```python
from build123d import *

# Parameters (mm, degrees)
REDONDEO1_R                            = 5
CORTAR_EXTRUIR1_REACH                  = 110.669
CORTAR_EXTRUIR1_END_RADIUS             = 20
CROQUIS2_W                             = 5
CROQUIS2_H                             = 30
CORTAR_EXTRUIR1_DIRECTION_2_REACH      = 110.669
CORTAR_EXTRUIR1_DIRECTION_2_END_RADIUS = 20
CORTAR_EXTRUIR3_REACH                  = 117.3
CORTAR_EXTRUIR3_END_RADIUS             = 9
CROQUIS3_R                             = 5


with BuildPart() as part:
    # Croquis1 → Revolución1 (revolve)
    with BuildSketch(Plane(origin=(0, 0, 0), x_dir=(1, 0, 0), z_dir=(0, 1, 0))):
        Polygon((25, 0), (42, 0), (42, 6), (31, 6), (31, 36), (20, 36), (20, 91), (9, 91), (9, 25), (25, 25), align=None)
    revolve(axis=Axis((0, 0, 3.677633668), (0, 0, -1)))

    # Redondeo1
    redondeo1_edges = [part.edges().sort_by_distance(p)[0] for p in [
        (-25, 0, -25),
        (-20, 0, -36),
        (-31, 0, -6),
    ]]
    fillet(redondeo1_edges, radius=REDONDEO1_R)

    # Cortar-Extruir1: up to this cylinder (the profile starts inside it)
    cortar_extruir1_end = Plane(origin=(0, 0, -66), z_dir=(0, 0, 1)) * Cylinder(CORTAR_EXTRUIR1_END_RADIUS, 262.338, mode=Mode.PRIVATE)
    # Croquis2 → Cortar-Extruir1 (cut, up to the surface)
    with BuildSketch(Plane(origin=(0, 0, 0), x_dir=(1, 0, 0), z_dir=(0, 1, 0)), mode=Mode.PRIVATE) as cortar_extruir1_sk1:
        with Locations((17.5, 66)):
            Rectangle(CROQUIS2_W, CROQUIS2_H)
    cortar_extruir1_tool1 = extrude(cortar_extruir1_sk1.sketch, amount=-CORTAR_EXTRUIR1_REACH, mode=Mode.PRIVATE) & cortar_extruir1_end
    cortar_extruir1 = cortar_extruir1_tool1.solids().sort_by_distance((17.5, 0, -66))[0]
    add(cortar_extruir1, mode=Mode.SUBTRACT)

    # Cortar-Extruir1 direction 2: up to this cylinder (the profile starts inside it)
    cortar_extruir1_direction_2_end = Plane(origin=(0, 0, -66), z_dir=(0, 0, 1)) * Cylinder(CORTAR_EXTRUIR1_DIRECTION_2_END_RADIUS, 262.338, mode=Mode.PRIVATE)
    # Croquis2 → Cortar-Extruir1 direction 2 (cut, up to the surface)
    with BuildSketch(Plane(origin=(0, 0, 0), x_dir=(1, 0, 0), z_dir=(0, 1, 0)), mode=Mode.PRIVATE) as cortar_extruir1_direction_2_sk1:
        with Locations((17.5, 66)):
            Rectangle(CROQUIS2_W, CROQUIS2_H)
    cortar_extruir1_direction_2_tool1 = extrude(cortar_extruir1_direction_2_sk1.sketch, amount=CORTAR_EXTRUIR1_DIRECTION_2_REACH, mode=Mode.PRIVATE) & cortar_extruir1_direction_2_end
    cortar_extruir1_direction_2 = cortar_extruir1_direction_2_tool1.solids().sort_by_distance((17.5, 0, -66))[0]
    add(cortar_extruir1_direction_2, mode=Mode.SUBTRACT)
    cortar_extruir1 = cortar_extruir1 + cortar_extruir1_direction_2  # both directions under the feature's name, for the pattern or mirror that repeats it

    # Cortar-Extruir3: up to this cylinder (the profile starts outside it)
    cortar_extruir3_end = Plane(origin=(0, 0, -66), z_dir=(0, 0, 1)) * Cylinder(CORTAR_EXTRUIR3_END_RADIUS, 253.6, mode=Mode.PRIVATE)
    # Croquis3 → Cortar-Extruir3 (cut, up to the surface)
    with BuildSketch(Plane(origin=(15, 0, 0), x_dir=(0, 0, -1), z_dir=(1, 0, 0)), mode=Mode.PRIVATE) as cortar_extruir3_sk1:
        with Locations((66, 0)):
            Circle(CROQUIS3_R)
    cortar_extruir3_tool1 = extrude(cortar_extruir3_sk1.sketch, amount=-CORTAR_EXTRUIR3_REACH, mode=Mode.PRIVATE) - cortar_extruir3_end
    cortar_extruir3 = cortar_extruir3_tool1.solids().sort_by_distance((15, 0, -66))[0]
    add(cortar_extruir3, mode=Mode.SUBTRACT)

    # Simetría2: Cortar-Extruir1, Cortar-Extruir3 across plane
    add(cortar_extruir1.mirror(Plane(origin=(0, 0, 0), x_dir=(0, 0, 1), z_dir=(1, 0, 0))), mode=Mode.SUBTRACT)
    add(cortar_extruir3.mirror(Plane(origin=(0, 0, 0), x_dir=(0, 0, 1), z_dir=(1, 0, 0))), mode=Mode.SUBTRACT)


solid = part.part
```
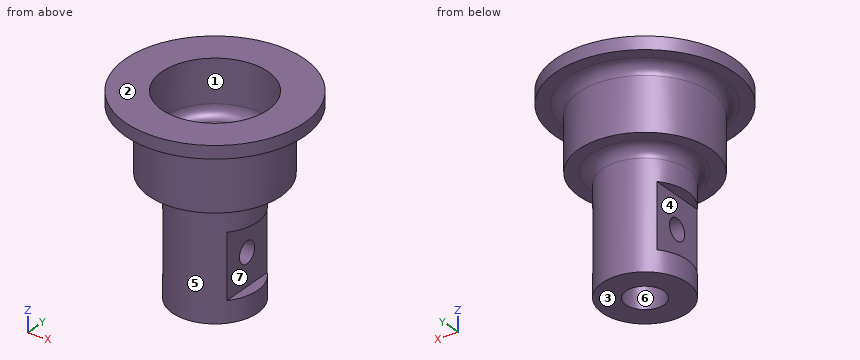
Design review of the part built by this model. Coordinates are the model's own, in mm. Face numbers are marked on the shaded views. A direction names the side the tool comes from. Coordinates: 2 decimals unless noted, no trailing zeros. Write each loop counter-clockwise with the first axis right and the second up, starting at its lowest first coordinate (ties: lowest second). Pieces come first, ordered by that corner, then holes.
1) To check wall thickness, follow L1, parallel to Z at x = -12, y = 0; L2, parallel to Z at x = 8.5, y = -25.5; L3, parallel to Z at x = -12.5, y = 10. State the ranges of each line that lie inside material, in increasing order.
2) Mouldability with a two-part tool opening along Z and no side actions: class the marked faces 1, 2, 3 and 4 as +Z half, -Z half, draft (parallel to the pull), parting line (faces both ways), or undercut.
3) Machinability: for the marked faces 5, 6 and 7, which of the approach directions +Z, -Z, +X, -X, +Y, -Y give a long, thin tool a straight path to every point of the face, cutting with its end or side? Answer none if there is none.
4) Add section D-D (z = -12.5). Write out the cut boundary in (x, y), plus the area to 3 significant figures.
5) Insertion check: pin 1 (1 mm diameter, centred on x = -7.5, y = -25.5, fed in from -Z); pin 2 (1 mm diameter, centred on x = 25.5, z = -17.5, fed in from -Y); pin 3 (12 mm diameter, centred on y = -9.5, z = -45, fed in from -X); pin 4 (9 mm diameter, centred on y = 0, z = -66, fed in from -X). Each pin has a flat end and moves straight along its axis. Give the tip position at first contact, or say it passes through.
6) Add section A-A (x = 0). Write out the cut boundary in (y, z), plus the area to 3 significant figures.
7) Add section B-B (z = -66). Write out the cut boundary in (x, y), plus the area to 3 significant figures.
8) Add section C-C (y = 0). State how many separate pieces and enclosed holes the cut face has, plus the area to 3 significant figures.
Check result:
1. L1: z = -91 to -71, -61 to -25
1. L2: z = -36 to 0
1. L3: z = -91 to -25
2. face 1: draft
2. face 2: +Z half
2. face 3: -Z half
2. face 4: undercut
3. face 5: -Z
3. face 6: +Z, -Z
3. face 7: +X, +Y, -Y
4. outline: circle Ø62 at (0, 0); hole circle Ø50 at (0, 0)
4. area: 1,060 mm2
5. pin 1: stops at z = -36
5. pin 2: stops at y = -18.33
5. pin 3: stops at x = -19.69
5. pin 4: passes through
6. outline: (-42, -6) - (-36, -6) arc R5 cw to (-31, -11) - (-31, -36) - (-25, -36) arc R5 cw to (-20, -41) - (-20, -91) - (-9, -91) - (-9, -25) - (-20, -25) arc R5 cw to (-25, -20) - (-25, 0) - (-42, 0) - close; (9, -91) - (20, -91) - (20, -41) arc R5 cw to (25, -36) - (31, -36) - (31, -11) arc R5 cw to (36, -6) - (42, -6) - (42, 0) - (25, 0) - (25, -20) arc R5 cw to (20, -25) - (9, -25) - close
6. area: 2,160 mm2
7. outline: (-15, -13.23) arc R20 ccw to (15, -13.23) - (15, -5) - (7.48, -5) arc R9 cw to (-7.48, -5) - (-15, -5) - close; (-15, 5) - (-7.48, 5) arc R9 cw to (7.48, 5) - (15, 5) - (15, 13.23) arc R20 ccw to (-15, 13.23) - close
7. area: 691 mm2
8. separate pieces: 4
8. enclosed holes: 0
8. area: 1,740 mm2
